Autodesk Inventor part; units mm, degrees
ref_plane "YZ Plane" through (0, 0, 0) normal (1, 0, 0) x (0, 1, 0)
ref_plane "XZ Plane" through (0, 0, 0) normal (0, 1, 0) x (-1, 0, 0)
ref_plane "XY Plane" through (0, 0, 0) normal (0, 0, 1) x (1, 0, 0)
sketch "Szkic1" plane through (0, 0, 0) normal (0, 1, 0) x (-1, 0, 0)
  line L0 (27.5, 28.9264) -> (-27.5, 28.9264)
  line L1 (-27.5, 28.9264) -> (-27.5, -66.0736)
  line L2 (-27.5, -66.0736) -> (27.5, -66.0736)
  line L3 (27.5, -66.0736) -> (27.5, 28.9264)
  line L4 (-12.5, -28.0736) -> (7.5, -28.0736)
  line L5 (7.5, -28.0736) -> (7.5, 8.9264)
  line L6 (7.5, 8.9264) -> (-12.5, 8.9264)
  line L7 (-12.5, 8.9264) -> (-12.5, -28.0736)
  point P0 (0, 0)
  point P1 (27.5, -18.5736)
  dimension "d0" = 55
  dimension "d1" = 95
  dimension "d3" = 20
  dimension "d4" = 37
  dimension "d5" = 38
  dimension "d6" = 40
extrude "Wyciągnięcie proste1" add sketch "Szkic1" along normal blind 12
sketch "Szkic2" plane through (0, 12, 0) normal (0, 1, 0) x (1, 0, 0)
  line L0 (-27.5, 66.0736) -> (-27.5, -28.9264)
  line L1 (-27.5, 66.0736) -> (12.5, 66.0736)
  line L2 (12.5, 66.0736) -> (12.5, 41.0736)
  line L3 (12.5, 41.0736) -> (-27.5, 41.0736)
  line L4 (-27.5, 41.0736) -> (-27.5, 66.0736)
  point P0 (0, 0)
  dimension "d9" = 40
  dimension "d10" = 25
extrude "Wyciągnięcie proste2" add sketch "Szkic2" along normal blind 76
sketch "Szkic3" plane through (0, 12, 0) normal (0, 1, 0) x (1, 0, 0)
  line L0 (-27.5, 66.0736) -> (-27.5, -28.9264)
  line L1 (12.5, 41.0736) -> (-27.5, 41.0736)
  line L2 (-27.5, -28.9264) -> (-15.5, -28.9264)
  line L3 (-15.5, -28.9264) -> (-15.5, 41.0736)
  line L4 (-15.5, 41.0736) -> (-27.5, 41.0736)
  line L5 (-27.5, 41.0736) -> (-27.5, -28.9264)
  point P0 (0, 0)
  dimension "d13" = 12
extrude "Wyciągnięcie proste3" add sketch "Szkic3" along normal blind 33
sketch "Szkic4" plane through (-15.5, 12, 28.9264) normal (1, 0, 0) x (0, 0, -1)
  line L0 (0, 0) -> (95, 0)
  point P0 (28.9264, -12)
  point P1 (15, 12)
  point P2 (52, 12)
  dimension "d16" = 12
  dimension "d17" = 12
sketch "Szkic5" plane through (-27.5, 88, -41.0736) normal (0, 0, 1) x (1, 0, 0)
  point P0 (27.5, -88)
  point P1 (20, -20)
hole "Otwór1" at (-15.5, 24, 13.9264) at (-15.5, 24, -23.0736) direction (-1, 0, 0) diameter 12 end through all
hole "Otwór2" at (-7.5, 68, -41.0736) direction (0, 0, -1) diameter 25 end through all
full round fillet "Zaokrąglenie pełne1" first side at (12.5, 62.6667, -49.4069) centre faces at (-14.1667, 88, -57.7402) second side at (-27.5, 44.3333, -57.7402)
fillet "Zaokrąglenie powierzchni1" radius 8 1 edges at (-21.5, 45, -41.0736)
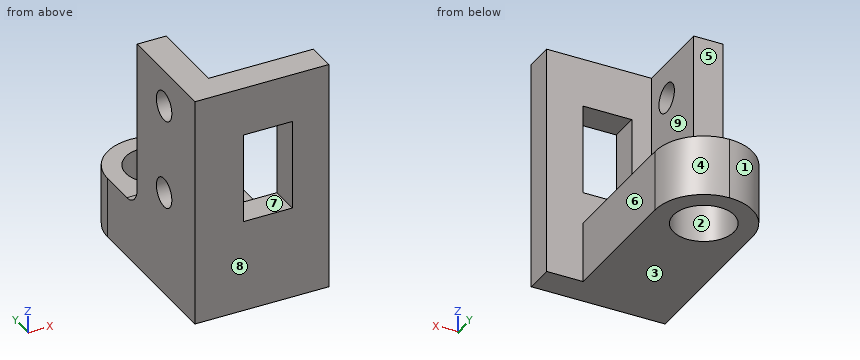
Input: part model. Units: mm. Frame: model coordinates. Face numbers are marked on the shaded views. A direction names the side the tool comes from. Round coordinates to 2 decimals unless told otherwise and drop trailing zeros. Order: outer loops, then holes, each group sorted by start corner. A loop starts at its lowest first (then second) coordinate and runs counter-clockwise, first axis right, second up.
1. Pin query (flat end, axial travel): P1, Ø7, axis at y = 24, z = 13.93, coming from the -X side; P2, Ø2, axis at x = 9, y = 65, coming from the +Z side; P3, Ø3.5, axis at x = -23.5, z = -13.5, coming from the +Y side; P4, Ø6, axis at x = -11, z = 5.5, coming from the +Y side. Return the tip coordinate at first contact, or that it passes through.
The answers:
P1: passes through
P2: stops at z = -41.07
P3: stops at y = 45
P4: stops at y = 12
2. Set-up query: the marked faces 5, 6, 7, 8 and 9. Return all of +Z, -Z, +X, -X, +Y, -Y with unobstructed straight access to the full face (end or side cutting, diameter ignored); none if empty.
The answers:
face 5: +Z, +X, -X, +Y
face 6: +Z, -Z, +X, +Y
face 7: +Y, -Y
face 8: +Z, -Z, +X, -X, -Y
face 9: +Z, +X, +Y
3. Material intervals for line 1 (Z direction, x = -18.25, y = 24); line 2 (X direction, y = 68, z = -60); line 3 (Y direction, x = 25, z = -45.5), sorted ascending.
The answers:
line 1: z = -66.07 to -29.07, -17.07 to 7.93, 19.93 to 28.93
line 2: x = -27.5 to -20, 5 to 12.5
line 3: y = 0 to 12
4. Mould query, pull axis X, two halves, no side actions, for the marked faces 1, 2, 3 and 4. Classes: released by +X, released by -X, zero draft, split by the parting line, or undercut.
The answers:
face 1: released by -X
face 2: undercut
face 3: zero draft
face 4: released by +X
5. Cut plane C-C, the plane z = 2.5. Output: boundary loops of the cut face in (x, y), then the cut area to 3 significant figures.
The answers:
outline: (-27.5, 0) - (-7.5, 0) - (-7.5, 12) - (-15.5, 12) - (-15.5, 45) - (-27.5, 45) - close; (12.5, 0) - (27.5, 0) - (27.5, 12) - (12.5, 12) - close
area: 816 mm2
6. Cut plane B-B, the plane x = -18.5. Output: boundary loops of the cut face in (y, z), then the cut area to 3 significant figures.
The answers:
outline: (0, -66.07) - (62.06, -66.07) - (62.06, -41.07) - (53, -41.07) arc R8 cw to (45, -33.07) - (45, 28.93) - (0, 28.93) - close; (73.94, -66.07) - (84.7, -66.07) - (84.7, -41.07) - (73.94, -41.07) - close; hole circle Ø12 at (24, -23.07); hole circle Ø12 at (24, 13.93)
area: 4,760 mm2
7. Cut plane D-D, the plane y = 63. Output: boundary loops of the cut face in (x, z).
The answers:
outline: (-27.5, -66.07) - (-18.96, -66.07) - (-18.96, -41.07) - (-27.5, -41.07) - close; (3.96, -66.07) - (12.5, -66.07) - (12.5, -41.07) - (3.96, -41.07) - close
8. Cut plane A-A, the plane y = 24. Output: boundary loops of the cut face in (x, z), then the cut area to 3 significant figures.
The answers:
outline: (-27.5, -66.07) - (12.5, -66.07) - (12.5, -41.07) - (-15.5, -41.07) - (-15.5, -29.07) - (-27.5, -29.07) - close; (-27.5, -17.07) - (-15.5, -17.07) - (-15.5, 7.93) - (-27.5, 7.93) - close; (-27.5, 19.93) - (-15.5, 19.93) - (-15.5, 28.93) - (-27.5, 28.93) - close
area: 1,550 mm2
